For this review, take the finished solid that the model builds, in its own axes (mm). Face numbers are marked on the shaded views. Round coordinates to 2 decimals unless told otherwise and drop trailing zeros. Loops run counter-clockwise (first coordinate to the right, second up) from the corner with the lowest first, then second, coordinate; pieces in that order, holes last.
1. Clearance check with a flat-ended pin moving along its axis: pin 1 Ø2 at (x, z) = (12.5, 1.5) entering from +Y. State where the tip first meets the part, or that it passes through.
2. Consider section C-C on z = 3.55. State the section outline as (x, y) points, then the cut area to 3 significant figures.
3. To check wall thickness, follow line 1 along Y through (x, z) = (-12, 1.8); line 2 along Y through (x, z) = (-11, 2.4) (3 decimals); line 3 along X through (y, z) = (3.25, 3.1). State the ranges of each line that lie inside material, in increasing order.
4. Consider section A-A on y = 5.5. State the section outline as (x, z) points.
5. Consider section B-B on x = 5.5. State the section outline as (y, z) points, then the cut area to 3 significant figures.
6. Draft analysis for pull direction Y (two halves, no side actions). For the marked faces 1, 2 and 3, state which applies: released by +Y, released by -Y, zero draft, split by the parting line, or undercut.
Autodesk Inventor part; units mm, degrees
ref_plane "YZ Plane" through (0, 0, 0) normal (1, 0, 0) x (0, 1, 0)
ref_plane "XZ Plane" through (0, 0, 0) normal (0, 1, 0) x (-1, 0, 0)
ref_plane "XY Plane" through (0, 0, 0) normal (0, 0, 1) x (1, 0, 0)
sketch "Sketch1" plane through (0, 0, 0) normal (0, 0, 1) x (1, 0, 0)
  circle A0 centre (66.3829, 0.6317) radius 13.7761
  line L0 (-12.0738, 8.6506) -> (65.3682, 14.3704)
  line L1 (-12.4772, -0.2842) -> (64.1342, -12.9596)
  line L2 (-12.0001, 7.6533) -> (-8.9346, 7.8797)
  arc A1 (64.2974, -11.973) -> (65.4418, 13.3731) centre (66.3829, 0.6317) ccw
  line L3 (64.2974, -11.973) -> (59.2137, -11.1319)
  arc A2 (-12.0001, 7.6533) -> (-12.314, 0.7024) centre (-11.7421, 4.1591) ccw
  line L4 (3.1814, -1.8614) -> (-12.314, 0.7024)
  line L5 (-8.9346, 7.8797) -> (60.3029, 12.9936)
  line L6 (59.2137, -11.1319) -> (3.1814, -1.8614)
  line L7 (60.3029, 12.9936) -> (65.4418, 13.3731)
  arc A3 (-9.1781, 7.8617) -> (-9.5222, 0.2405) centre (-11.7421, 4.1591) ccw
  arc A4 (-9.5222, 0.2405) -> (-9.1781, 7.8617) centre (-11.7421, 4.1591) ccw
  point P0 (0, 0)
  dimension "d0" = 1
extrude "Extrusion2" add sketch "Sketch1" along normal blind 6 contours A0 L3 A1 L7 | A0 L5 L2 A3 L0 | L1 A3 L4 L6 A0 | A3 L2 A2 L4 picked at (66.3473, -12.7206)
properties part number "Belt"
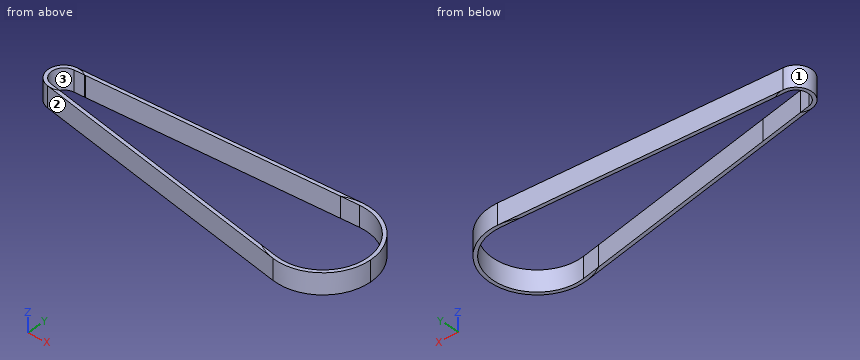
Resolved:
1. pin 1: stops at y = 10.54
2. outline: (-12.48, -0.28) - (64.13, -12.96) arc R13.78 ccw (long way) to (65.37, 14.37) - (-12.07, 8.65) arc R4.5 ccw to start; hole (-12.31, 0.7) - (3.18, -1.86) - (59.21, -11.13) - (64.3, -11.97) arc R12.78 ccw (long way) to (65.44, 13.37) - (60.3, 12.99) - (-8.93, 7.88) - (-12, 7.65) arc R3.5 ccw to start
2. area: 212 mm2
3. line 1: y = -0.36 to 0.65, 7.65 to 8.66
3. line 2: y = -0.529 to 0.485, 7.727 to 8.73
3. line 3: x = -16.15 to -15.13, 78.89 to 79.91
4. outline: (-16.04, 0) - (-14.98, 0) - (-14.98, 6) - (-16.04, 6) - close; (78.2, 0) - (79.27, 0) - (79.27, 6) - (78.2, 6) - close
5. outline: (-3.26, 0) - (-2.25, 0) - (-2.25, 6) - (-3.26, 6) - close; (8.95, 0) - (9.95, 0) - (9.95, 6) - (8.95, 6) - close
5. area: 12.1 mm2
6. face 1: split by the parting line
6. face 2: released by -Y
6. face 3: undercut
